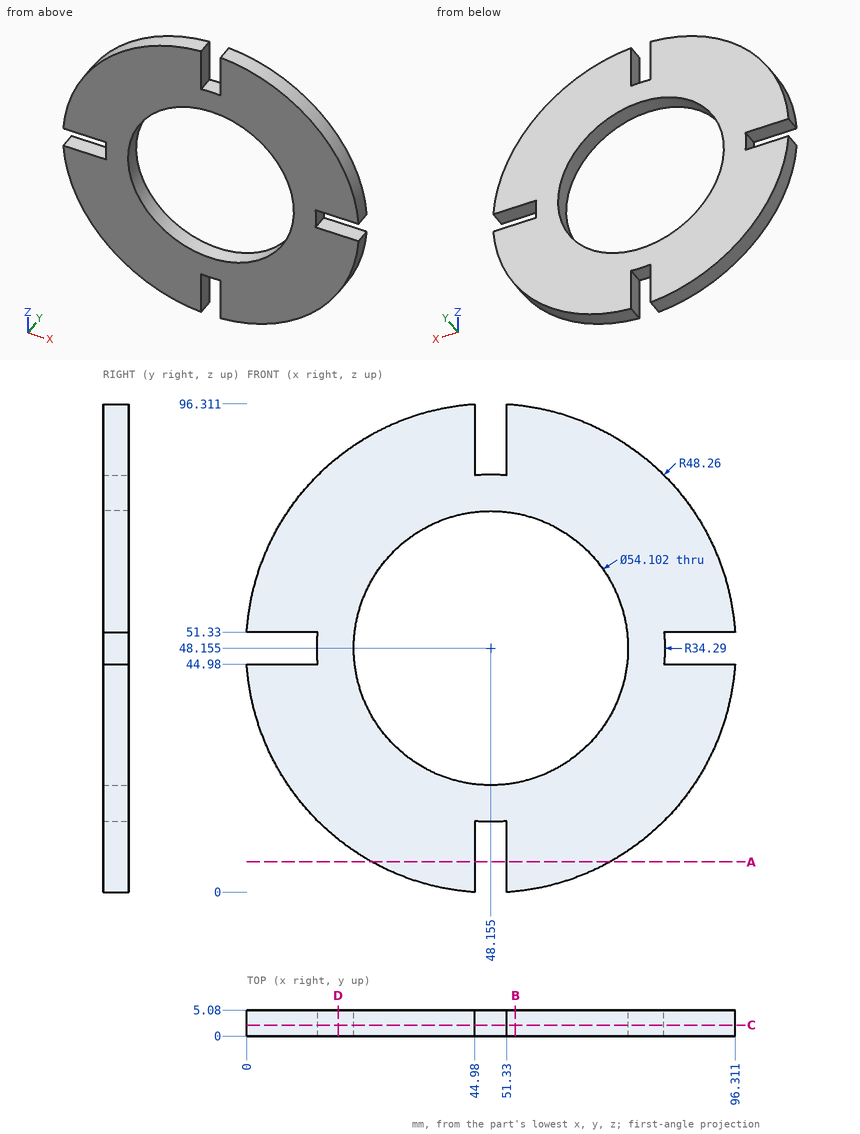
The figure shows three views and two pictorial views of one solid part (mm, origin at its lowest corner). Answer the questions. Round coordinates to 2 decimals unless told otherwise and drop trailing zeros. Write each loop counter-clockwise with the first axis right and the second up, starting at its lowest first coordinate (ties: lowest second). Pieces come first, ordered by that corner, then holes. Notation, with made-up numbers: M 51.25,50.5 L 80.25,50.5 A28 cw 80.25,84.5 Z; hole C 34,8.25 d9. An arc over 180 degrees is marked long. Use a Markdown table: item, result.
1) Straight lines are drawn through the part: line 1 along X through (y, z) = (3.4, 46); line 2 along X through (y, z) = (3.7, 44) (1 decimal); line 3 along Z through (x, y) = (47, 2.85) (1 decimal). For each, find the intervals that lie inside material, in ascending order. Write a range as [from, to].
Answers follow:
| item | result |
|---|---|
| line 1 | x = [13.93, 21.19], [75.12, 82.38] |
| line 2 | x = [0.1, 21.4], [74.9, 96.2] |
| line 3 | z = [13.9, 21.1], [75.2, 82.4] |
2) The part is cut by section D-D (x = 18). Write down the section's boundary in (y, z).
Answers follow:
| item | result |
|---|---|
| outline | M 0,10.48 L 5.08,10.48 L 5.08,85.83 L 0,85.83 Z |
3) The part is cut by section A-A (z = 6). Write down the section's boundary in (x, y).
Answers follow:
| item | result |
|---|---|
| outline | M 24.66,0 L 44.98,0 L 44.98,5.08 L 24.66,5.08 Z; M 51.33,0 L 71.65,0 L 71.65,5.08 L 51.33,5.08 Z |
4) Flat-ended cylindrical pins translate along their axes: pin 1 (1.5 mm diameter, centred on x = 14, y = 0.5, fed in from -Z) (1 decimal); pin 2 (2.5 mm diameter, centred on y = 4, z = 4.5, fed in from -X) (1 decimal); pin 3 (2.5 mm diameter, centred on x = 10, y = 2, fed in from -Z). Find the tip coordinate at first contact, or state that the pin passes through.
Answers follow:
| item | result |
|---|---|
| pin 1 | stops at z = 13.3 |
| pin 2 | stops at x = 25.1 |
| pin 3 | stops at z = 17.06 |
5) The part is cut by section B-B (x = 53). Write down the section's boundary in (y, z).
Answers follow:
| item | result |
|---|---|
| outline | M 0,0.14 L 5.08,0.14 L 5.08,21.54 L 0,21.54 Z; M 0,74.77 L 5.08,74.77 L 5.08,96.17 L 0,96.17 Z |
6) The part is cut by section C-C (y = 2.15). Write down the section's boundary in (x, z) (1 decimal), plus the area to 3 significant figures.
Answers follow:
| item | result |
|---|---|
| outline | M 0,45 A48.3 ccw 45,0 L 45,14 A34.3 ccw 51.3,14 L 51.3,0 A48.3 ccw 96.3,45 L 82.3,45 A34.3 ccw 82.3,51.3 L 96.3,51.3 A48.3 ccw 51.3,96.3 L 51.3,82.3 A34.3 ccw 45,82.3 L 45,96.3 A48.3 ccw 0,51.3 L 14,51.3 A34.3 ccw 14,45 Z; hole C 48.2,48.2 d54.1 |
| area | 4,660 mm2 |
